Can you work these out from the model? Positions are in its coordinate system, mm. A direction names the side the tool comes from. Coordinates: 2 decimals unless noted, no trailing zeros. Order: outer loops, then holes, each group sorted by start corner. A loop starts at its lowest first (then second) coordinate and runs counter-clockwise, first axis right, second up. Notation, with made-up numbers: M -24.75,30.5 L -17.75,30.5 A38 cw -17.75,69.5 Z; hole C 70,74.5 d4. An arc over 180 degrees is marked long. Answer as CSV lines item,"result". Start each with the question number.
1. I need wall thicknesses on line 1 along Z through (x, y) = (0.4, -4.75); line 2 along Y through (x, z) = (1, 2.8); line 3 along Y through (x, z) = (2, 3). Which ranges of each line are inside material? Lowest first, please. Write a range as from..to.
2. If we section it at B-B (y = -3): List the corners of the cut face in (x, z) for me, plus the area to 3 significant figures.
3. On a 3-axis mill with a long thin cutter (end or side, diameter ignored), from which of +Z, -Z, +X, -X, +Y, -Y can I reach the whole of each face in a straight line? I mean faces 4 (the face through (3, -3, 4.3)), 5 (the face through (4.008, -4.938, 3.387)). Say none if no direction works.
4. If we section it at D-D (y = -5.45): List the corners of the cut face in (x, z) for me.
5. If we section it at A-A (x = 3): List the corners of the cut face in (y, z) for me, plus the area to 3 significant figures.
6. If we section it at C-C (z = 4): List the corners of the cut face in (x, y) for me.
7. If we mould it in two halves opening along Y, with no side actions, what happens to faces 1 (the face through (6, -3, 1)), 2 (the face through (3, -6, 1)), 3 (the face through (4.3, -1, 2.5))? For each: released by +Y, released by -Y, zero draft, split by the parting line, or undercut.
```python
from build123d import *

# Parameters (mm, degrees)
F0_W     = 6
F0_H     = 6
F1_DEPTH = 2.5
F2_R     = 2.18397174
F3_DEPTH = 1.8
F2_R_2   = 0.2032
F4_DEPTH = 0.2


with BuildPart() as f1:
    # F0 (on Top) → F1 (new body)
    with BuildSketch(Plane.XY):
        with Locations((3, -3)):
            Rectangle(F0_W, F0_H)
    extrude(amount=F1_DEPTH)

    # F2 (on face) → F3 (join)
    with BuildSketch(Plane.XY.offset(2.5)):
        with Locations((3, -3)):
            Circle(F2_R)
    extrude(amount=F3_DEPTH)

    # F2 (on face) → F4 (join)
    with BuildSketch(Plane.XY.offset(2.5)):
        with BuildLine():
            ThreePointArc((0.6254458211, -0.4234319816), (0.5007393311, -0.23679553), (0.2805866258, -0.2805866258))
            ThreePointArc((0.2805866258, -0.2805866258), (0.2805866258, -0.5662773374), (0.5662773374, -0.5662773374))
            ThreePointArc((0.5662773374, -0.5662773374), (0.6100684332, -0.5007393311), (0.6254458211, -0.4234319816))
        make_face()
        with BuildLine():
            ThreePointArc((5.7797680184, -5.5765680184), (5.3888356974, -5.498806745), (5.7202521163, -5.7202521163))
            ThreePointArc((5.7202521163, -5.7202521163), (5.7643003394, -5.6543292919), (5.7797680184, -5.5765680184))
        make_face()
        with BuildLine():
            ThreePointArc((5.7797680184, -0.4234319816), (5.7643003394, -0.3456707081), (5.7202521163, -0.2797478837))
            ThreePointArc((5.7202521163, -0.2797478837), (5.3888356974, -0.501193255), (5.7797680184, -0.4234319816))
        make_face()
        with Locations((0.4234319816, -5.5765680184)):
            Circle(F2_R_2)
    extrude(amount=F4_DEPTH)


solid = f1.part
```
Solved:
1,line 1,"0..2.5"
1,line 2,"-3.88..-2.12"
1,line 3,"-4.94..-1.06"
2,outline,"M 0,0 L 6,0 L 6,2.5 L 5.18,2.5 L 5.18,4.3 L 0.82,4.3 L 0.82,2.5 L 0,2.5 Z"
2,area,"22.9 mm²"
3,face 4,"+Z, +X, -X, +Y, -Y"
3,face 5,"+Z"
4,outline,"M 0,0 L 6,0 L 6,2.5 L 5.74,2.5 L 5.74,2.7 L 5.42,2.7 L 5.42,2.5 L 0.58,2.5 L 0.58,2.7 L 0.26,2.7 L 0.26,2.5 L 0,2.5 Z"
5,outline,"M -6,0 L 0,0 L 0,2.5 L -0.82,2.5 L -0.82,4.3 L -5.18,4.3 L -5.18,2.5 L -6,2.5 Z"
5,area,"22.9 mm²"
6,outline,"C 3,-3 d4.37"
7,face 1,"zero draft"
7,face 2,"released by -Y"
7,face 3,"undercut"
